Input: part model. Units: mm. Frame: model coordinates. Face numbers are marked on the shaded views. A direction names the side the tool comes from. Round coordinates to 2 decimals unless told otherwise and drop trailing zeros. Loops run counter-clockwise (first coordinate to the right, second up) from the corner with the lowest first, then second, coordinate; pieces in that order, holes last.
1) Section B-B, the plane y = -33. Return loops of the section in (x, z), and give its area (4 significant figures).
2) First-contact query: pin 1 (6 mm diameter, centred on x = 8, z = 3, fed in from +Y); pin 2 (5.5 mm diameter, centred on x = 6, y = -3.5, fed in from +Z); pin 3 (2 mm diameter, centred on x = -24.5, z = 6, fed in from -Y); pin 4 (5 mm diameter, centred on y = -25.5, z = 20.5, fed in from +X). Flat tips, straight axial feed; report the tip coordinate or a pass-through.
3) Section D-D, the plane x = -2. Return loops of the section in (y, z), and give its area (3 significant figures).
4) Section C-C, the plane z = 14. Return loops of the section in (x, y).
5) Access query for the marked faces 1 and 2. Directions: +Z, -Z, +X, -X, +Y, -Y. A direction counts if a zero-diameter tool reaches every point of the face in a straight line with its end or side. Return the directions, or none.
6) Ray query, line 1 along Z through (x, y) = (3.05, -2.15); line 2 along Z through (x, y) = (-77, -19); line 3 along X through (y, z) = (-12, 20). Return the intervals inside material, ascending.
7) Section A-A, the plane x = -54. Return loops of the section in (y, z), and give its area (3 significant figures).
from build123d import *

# Parameters (mm, degrees)
RESSALTO_EXTRUS_O1_DEPTH = 5
ESBO_O2_W                = 50
ESBO_O2_H                = 17.09
RESSALTO_EXTRUS_O2_DEPTH = 32
ESBO_O3_R                = 0.94
CORTE_EXTRUS_O1_DEPTH    = 38
CORTE_EXTRUS_O2_DEPTH    = 2


with BuildPart() as part:
    # Esboço1 → Ressalto-extrusão1 (new body)
    with BuildSketch(Plane(origin=(0, 0, 0), x_dir=(1, 0, 0), z_dir=(0, 1, 0))):
        with BuildLine():
            ThreePointArc((-12.5, -10), (-21.738795325, -3.826834324), (-19.571067812, 7.071067812))
            Line((-19.571067812, 7.071067812), (-37.248737342, -10.606601718))
            Line((-37.248737342, -10.606601718), (-87.248737342, -10.606601718))
            Line((-87.248737342, -10.606601718), (-87.248737342, -27.696601718))
            Line((-87.248737342, -27.696601718), (-30.196551164, -27.696601718))
            ThreePointArc((-30.196551164, -27.696601718), (-26.357368714, -26.930272609), (-23.106601718, -24.748737342))
            Line((-23.106601718, -24.748737342), (-8.357864376, -10))
            Line((-8.357864376, -10), (-12.5, -10))
        make_face()
        with BuildLine():
            Line((-12.5, -10), (12.5, -10))
            ThreePointArc((12.5, -10), (22.5, 0), (12.5, 10))
            Line((12.5, 10), (-12.5, 10))
            ThreePointArc((-12.5, 10), (-22.5, 0), (-12.5, -10))
        make_face()
    extrude(amount=-RESSALTO_EXTRUS_O1_DEPTH)

    # Esboço2 → Ressalto-extrusão2 (add)
    with BuildSketch(Plane.XZ.offset(5)):
        with Locations((-62.248737342, 19.151601718)):
            Rectangle(ESBO_O2_W, ESBO_O2_H)
    extrude(amount=RESSALTO_EXTRUS_O2_DEPTH)

    # Esboço3 → Corte-extrusão1 (cut, through all)
    with BuildSketch(Plane(origin=(0, 0, 0), x_dir=(1, 0, 0), z_dir=(0, 1, 0))):
        with Locations((3.05, 0)):
            Circle(ESBO_O3_R)
    extrude(amount=-CORTE_EXTRUS_O1_DEPTH, mode=Mode.SUBTRACT)

    # Esboço6 → Corte-extrusão2 (cut)
    with BuildSketch(Plane(origin=(0, -5, 0), x_dir=(1, 0, 0), z_dir=(0, 1, 0))):
        with BuildLine():
            Line((-11, 2), (0.840927797, 2.65))
            ThreePointArc((0.840927797, 2.65), (3.05, 3.45), (5.259072203, 2.65))
            Line((5.259072203, 2.65), (17.1, 2))
            ThreePointArc((17.1, 2), (19.1, 0), (17.1, -2))
            Line((17.1, -2), (5.259072203, -2.65))
            ThreePointArc((5.259072203, -2.65), (3.05, -3.45), (0.840927797, -2.65))
            Line((0.840927797, -2.65), (-11, -2))
            ThreePointArc((-11, -2), (-13, 0), (-11, 2))
        make_face()
    extrude(amount=CORTE_EXTRUS_O2_DEPTH, mode=Mode.SUBTRACT)


solid = part.part
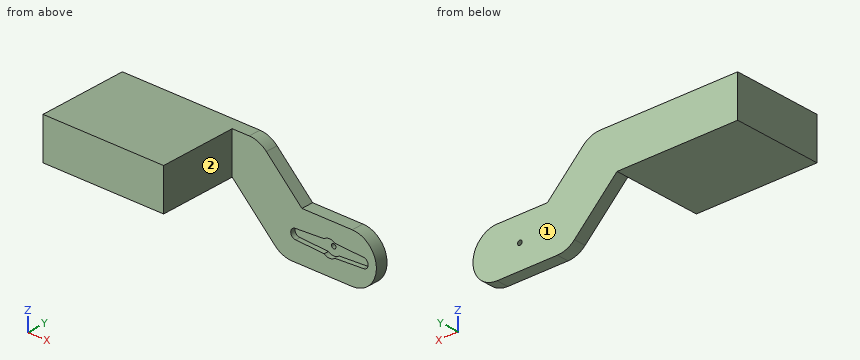
Final values:
1. outline: (-87.25, 10.61) - (-37.25, 10.61) - (-37.25, 27.7) - (-87.25, 27.7) - close
1. area: 854.5 mm2
2. pin 1: stops at y = 0
2. pin 2: stops at z = 10
2. pin 3: stops at y = -5
2. pin 4: stops at x = -37.25
3. outline: (-5, -10) - (0, -10) - (0, 10) - (-5, 10) - (-5, 2.49) - (-3, 2.49) - (-3, -2.49) - (-5, -2.49) - close
3. area: 90.0 mm2
4. outline: (-87.25, -37) - (-37.25, -37) - (-37.25, -5) - (-12.36, -5) - (-12.36, 0) - (-87.25, 0) - close
5. face 1: +Z, -Z, +X, -X, +Y
5. face 2: +Z, -Z, +X, -Y
6. line 1: z = -10 to -0.94, 0.94 to 10
6. line 2: z = 10.61 to 27.7
6. line 3: x = -87.25 to -37.25
7. outline: (-37, 10.61) - (0, 10.61) - (0, 27.7) - (-37, 27.7) - close
7. area: 632 mm2
